Autodesk Fusion 360 part; units mm, degrees
sketch "Sketch1" plane through (0, 0, 0) normal (0, 0, 1) x (1, 0, 0)
  circle A0 centre (0, 0) radius 2.75
  line L0 (0.675, -2.1) -> (-0.675, -2.1)
  line L1 (-0.675, 0.975) -> (-0.675, 2.1)
  line L2 (-0.675, 2.1) -> (0.675, 2.1)
  line L3 (0.675, -0.975) -> (0.675, -2.1)
  line L4 (0.675, -2.1) -> (-0.675, 2.1) construction
  line L5 (-0.675, -2.1) -> (0.675, 2.1) construction
  line L6 (2.1, -0.675) -> (0.975, -0.675)
  line L7 (-2.1, -0.675) -> (-2.1, 0.675)
  line L8 (0.975, 0.675) -> (2.1, 0.675)
  line L9 (2.1, 0.675) -> (2.1, -0.675)
  line L10 (2.1, -0.675) -> (-2.1, 0.675) construction
  line L11 (-2.1, -0.675) -> (2.1, 0.675) construction
  arc A1 (0.975, -0.675) -> (0.675, -0.975) centre (0.975, -0.975) ccw
  line L12 (0.675, 2.1) -> (0.675, 0.975)
  arc A2 (0.675, 0.975) -> (0.975, 0.675) centre (0.975, 0.975) ccw
  line L13 (-2.1, 0.675) -> (-0.975, 0.675)
  line L14 (-2.1, -0.675) -> (-0.975, -0.675)
  arc A3 (-0.975, 0.675) -> (-0.675, 0.975) centre (-0.975, 0.975) ccw
  line L15 (-0.675, -0.975) -> (-0.675, -2.1)
  arc A4 (-0.675, -0.975) -> (-0.975, -0.675) centre (-0.975, -0.975) ccw
  point P0 (0.675, -0.675)
  dimension "d1" = 5.5
  dimension "d2" = 1.35
  dimension "d3" = 4.2
  dimension "d4" = 4.2
  dimension "d5" = 1.35
  dimension "d6" = 0.3
  dimension "d7" = 0.3
  dimension "d8" = 0.3
  dimension "d9" = 0.3
extrude "Extrude1" add sketch "Sketch1" along normal blind 3.3
sketch "Sketch2" plane through (0, 0, 0) normal (0, 0, -1) x (1, 0, 0)
  line L0 (-2.1, 0.675) -> (-0.975, 0.675)
  arc A0 (-0.975, 0.675) -> (-0.675, 0.975) centre (-0.975, 0.975) ccw
  line L1 (-0.675, 0.975) -> (-0.675, 2.1)
  line L2 (-0.675, 2.1) -> (0.675, 2.1)
  line L3 (0.675, 2.1) -> (0.675, 0.975)
  arc A1 (0.675, 0.975) -> (0.975, 0.675) centre (0.975, 0.975) ccw
  line L4 (0.975, 0.675) -> (2.1, 0.675)
  line L5 (2.1, 0.675) -> (2.1, -0.675)
  line L6 (2.1, -0.675) -> (0.975, -0.675)
  arc A2 (0.975, -0.675) -> (0.675, -0.975) centre (0.975, -0.975) ccw
  line L7 (0.675, -0.975) -> (0.675, -2.1)
  line L8 (0.675, -2.1) -> (-0.675, -2.1)
  line L9 (-0.675, -2.1) -> (-0.675, -0.975)
  arc A3 (-0.675, -0.975) -> (-0.975, -0.675) centre (-0.975, -0.975) ccw
  line L10 (-0.975, -0.675) -> (-2.1, -0.675)
  line L11 (-2.1, -0.675) -> (-2.1, 0.675)
  circle A4 centre (0, 0) radius 2.75
  line L12 (4, 4) -> (-4, 4)
  line L13 (-4, 4) -> (-4, -4)
  line L14 (-4, -4) -> (4, -4)
  line L15 (4, -4) -> (4, 4)
  line L16 (4, 4) -> (-4, -4) construction
  line L17 (-4, 4) -> (4, -4) construction
  dimension "d12" = 8
  dimension "d13" = 8
extrude "Extrude2" add sketch "Sketch2" along normal blind 1 contours L0 A0 L1 L2 L3 A1 L4 L5 L6 A2 L7 L8 L9 A3 L10 L11 | A4 | L12 L13 L14 L15
fillet "Fillet1" radius 0.25 1 edges at (-2.5639, -0.9944, 0)
fillet "Fillet2" radius 0.2 1 edges at (-2.5639, -0.9944, 3.3)
fillet "Fillet3" radius 0.2 16 edges at (1.5375, -0.675, 3.3) (0.7629, -0.7629, 3.3) (0.675, -1.5375, 3.3) (2.1, 0, 3.3) (0.675, 1.5375, 3.3) (0.7629, 0.7629, 3.3) (1.5375, 0.675, 3.3) (0, 2.1, 3.3) (-1.5375, 0.675, 3.3) (-0.7629, 0.7629, 3.3) (-0.675, 1.5375, 3.3) (-2.1, 0, 3.3) (-0.675, -1.5375, 3.3) (-0.7629, -0.7629, 3.3) (-1.5375, -0.675, 3.3) (0, -2.1, 3.3)
equation "d2 = cross_thickness"
equation "d3 = cross_xy"
equation "d4 = cross_xy"
equation "d5 = cross_thickness"
equation "d10 = stem_height"
equation "cross_xy = 4.20 mm"
equation "cross_thickness = 1.35 mm"
equation "stem_height = 3.3 mm"
Part model, mm, in its own coordinate system. A direction names the side the tool comes from. Give positions to 0.01 mm unless a question says otherwise; leave off trailing zeros. Write each loop counter-clockwise with the first axis right and the second up, starting at its lowest first coordinate (ties: lowest second). Pieces come first, ordered by that corner, then holes. Notation, with made-up numbers: (49.25, 63) -> (97.25, 63) arc R24 ccw to (97.25, 73) -> close; hole circle Ø8 at (46.5, 29). An arc over 180 degrees is marked (long way). Put each result on its own line as item: value. Start each with the question number.
Item 1: Cut at D-D (x = 3.5). List the corners of the cut face in (y, z).
Item 2: Cut at A-A (z = 1.85). List the corners of the cut face in (x, y) (3 decimals).
Item 3: Which spindle directions (+Z, -Z, +X, -X, +Y, -Y) get a long thin tool onto all of the face, cutting with end or side? Do faces 1 (the face through (0.1, -4, -0.5)), 2 (the face through (-1.5, -0.675, 1.5)). Say none if no direction does.
Item 4: Pin check, flat tips, straight feed: pin 1 Ø0.7 at (x, z) = (0, 1.5) entering from +Y; pin 2 Ø0.6 at (x, z) = (2, 2) entering from -Y; pin 3 Ø0.6 at (x, z) = (1.5, 1) entering from +Y. Stop position of each tip, or through.
Item 5: Pull direction X, two halves, no side cores. Call faces 3 (the face through (2, -3, 0)), 4 (the face through (-0.675, 1.5, 1.5)), 5 (the face through (0.675, 1.5, 1.5)), 6 (the face through (-0.596, 2.685, 1.655)): pulls with the +X half, pulls with the -X half, needs draft (parallel to the pull), parting line crosses it, or undercut.
Item 6: Cut at B-B (x = 0). List the corners of the cut face in (y, z), then the cut area to 3 significant figures.
Item 7: Wall check: L1, parallel to Y at x = 0, z = 1.05; L2, parallel to Z at x = -1.25, y = 0.25; L3, parallel to X at y = 1.25, z = 1.4 (3 decimals). Give the ranges that are in metal, low to high. Write a range as [from, to].
Answer list:
1. outline: (-4, -1) -> (4, -1) -> (4, 0) -> (-4, 0) -> close
2. outline: circle Ø5.5 at (0, 0); hole (-2.1, -0.675) -> (-0.975, -0.675) arc R0.3 cw to (-0.675, -0.975) -> (-0.675, -2.1) -> (0.675, -2.1) -> (0.675, -0.975) arc R0.3 cw to (0.975, -0.675) -> (2.1, -0.675) -> (2.1, 0.675) -> (0.975, 0.675) arc R0.3 cw to (0.675, 0.975) -> (0.675, 2.1) -> (-0.675, 2.1) -> (-0.675, 0.975) arc R0.3 cw to (-0.975, 0.675) -> (-2.1, 0.675) -> close
3. face 1: +Z, -Z, +X, -X, -Y
3. face 2: +Z
4. pin 1: stops at y = 2.75
4. pin 2: stops at y = -2.16
4. pin 3: stops at y = 2.47
5. face 3: needs draft
5. face 4: undercut
5. face 5: undercut
5. face 6: parting line crosses it
6. outline: (-4, -1) -> (4, -1) -> (4, 0) -> (3, 0) arc R0.25 cw to (2.75, 0.25) -> (2.75, 3.1) arc R0.2 ccw to (2.55, 3.3) -> (2.3, 3.3) arc R0.2 ccw to (2.1, 3.1) -> (2.1, 0) -> (-2.1, 0) -> (-2.1, 3.1) arc R0.2 ccw to (-2.3, 3.3) -> (-2.55, 3.3) arc R0.2 ccw to (-2.75, 3.1) -> (-2.75, 0.25) arc R0.25 cw to (-3, 0) -> (-4, 0) -> close
6. area: 12.3 mm2
7. L1: y = [-2.75, -2.1], [2.1, 2.75]
7. L2: z = [-1, 0]
7. L3: x = [-2.449, -0.675], [0.675, 2.449]
